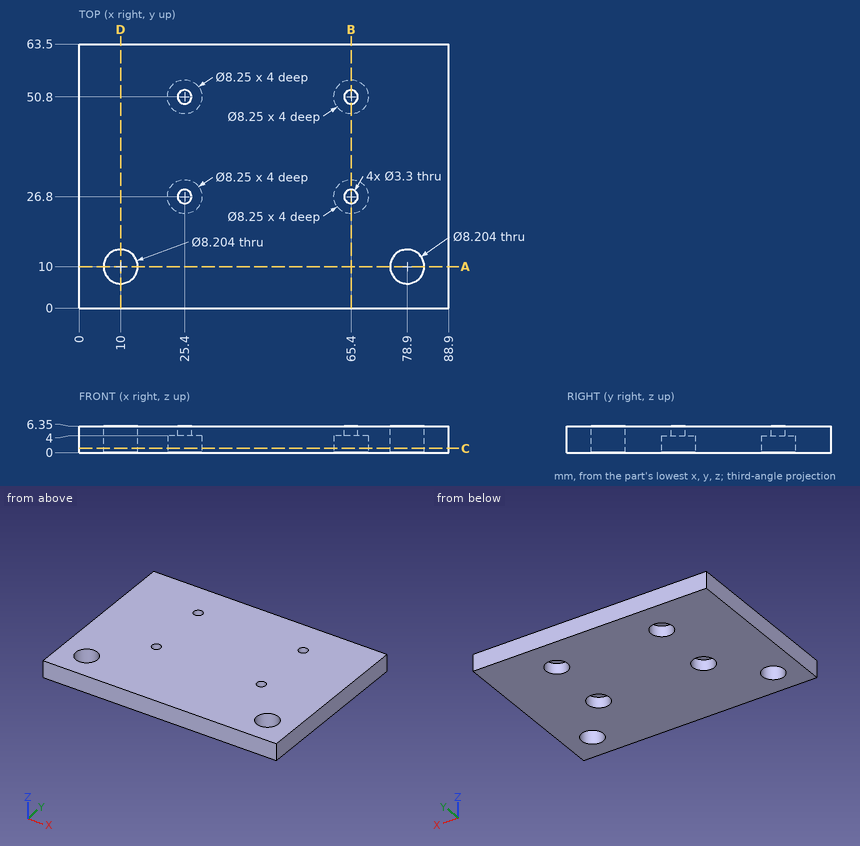
Verification items for this drawing (mm, ordinates from the low corner). Give positions to 0.01 mm unless a question says otherwise; leave off trailing zeros. Loops run counter-clockwise (first coordinate to the right, second up) from the corner with the lowest first, then second, coordinate; pieces in that order, holes last. Notation, with made-up numbers: M 72,-22.5 L 115,-22.5 A24 ccw 115,-11.5 Z; hole C 40.25,22 d7. An arc over 180 degrees is marked long. Answer as a JSON object with one key per item and string values. Group by question number.
Q1. Cross-section at A-A on y = 10. Record the cut outline in (x, z), then the cut area to 3 significant figures.
Q2. Cross-section at C-C on z = 1. Give the number of separate pieces and of enclosed holes in the cut face, then the cut area to 3 significant figures.
Q3. Cross-section at D-D on x = 10. Record the cut outline in (y, z), then the cut area to 3 significant figures.
Q4. Material ranges on line 1 along Y through (x, z) = (65.4, 2.2) (3 decimals); line 2 along X through (y, z) = (26.5, 2.25); line 3 along X through (y, z) = (27, 5.5), recorded low to high. Write a range as [from, to].
Q5. Go/stop test with a flat-tipped pin: P1, Ø5.5, axis at x = 25.4, y = 50.8, coming from the -Z side. Record where the tip stops, or that it passes through.
Q6. Cross-section at B-B on x = 65.4. Record the cut outline in (y, z) (3 decimals), then the cut area to 3 significant figures.
Evaluation:
{
 "1": {"outline": "M 0,0 L 5.9,0 L 5.9,6.35 L 0,6.35 Z; M 14.1,0 L 74.8,0 L 74.8,6.35 L 14.1,6.35 Z; M 83,0 L 88.9,0 L 88.9,6.35 L 83,6.35 Z", "area": "460 mm2"},
 "2": {"separate pieces": "1", "enclosed holes": "6", "area": "5,330 mm2"},
 "3": {"outline": "M 0,0 L 5.9,0 L 5.9,6.35 L 0,6.35 Z; M 14.1,0 L 63.5,0 L 63.5,6.35 L 14.1,6.35 Z", "area": "351 mm2"},
 "4": {"line 1": "y = [0, 22.675], [30.925, 46.675], [54.925, 63.5]", "line 2": "x = [0, 21.29], [29.51, 61.29], [69.51, 88.9]", "line 3": "x = [0, 23.76], [27.04, 63.76], [67.04, 88.9]"},
 "5": {"P1": "stops at z = 4"},
 "6": {"outline": "M 0,0 L 22.675,0 L 22.675,4 L 25.15,4 L 25.15,6.35 L 0,6.35 Z; M 28.45,4 L 30.925,4 L 30.925,0 L 46.675,0 L 46.675,4 L 49.15,4 L 49.15,6.35 L 28.45,6.35 Z; M 52.45,4 L 54.925,4 L 54.925,0 L 63.5,0 L 63.5,6.35 L 52.45,6.35 Z", "area": "322 mm2"}
}
